Autodesk Inventor part; units mm, degrees
ref_plane "YZ Plane" through (0, 0, 0) normal (1, 0, 0) x (0, 1, 0)
ref_plane "XZ Plane" through (0, 0, 0) normal (0, 1, 0) x (-1, 0, 0)
ref_plane "XY Plane" through (0, 0, 0) normal (0, 0, 1) x (1, 0, 0)
sketch "Sketch1" plane through (0, 0, 0) normal (0, 0, 1) x (1, 0, 0)
  circle A0 centre (0, 0) radius 38.1
  circle A1 centre (0, 0) radius 31.75
  line L0 (-84.6709, -3.175) -> (-84.6709, 3.175)
  line L1 (84.6709, 3.175) -> (84.6709, -3.175)
  line L2 (84.6709, -3.175) -> (-84.6709, 3.175) construction
  line L3 (-84.6709, -3.175) -> (84.6709, 3.175) construction
  line L4 (84.6709, -3.175) -> (37.9675, -3.175)
  line L5 (-37.9675, -3.175) -> (-84.6709, -3.175)
  line L6 (-84.6709, 3.175) -> (-37.9675, 3.175)
  line L7 (37.9675, 3.175) -> (84.6709, 3.175)
  line L8 (-84.6709, 22.225) -> (-77.0509, 22.225)
  line L9 (-77.0509, 22.225) -> (-77.0509, -22.225)
  line L10 (-77.0509, -22.225) -> (-84.6709, -22.225)
  line L11 (-84.6709, -22.225) -> (-84.6709, 22.225)
  line L12 (0, 31.75) -> (0, -31.75) construction
  line L13 (84.6709, 22.225) -> (77.0509, 22.225)
  line L14 (77.0509, 22.225) -> (77.0509, -22.225)
  line L15 (77.0509, -22.225) -> (84.6709, -22.225)
  line L16 (84.6709, -22.225) -> (84.6709, 22.225)
  dimension "d0" = 76.2
  dimension "d1" = 6.35
  dimension "d2" = 169.3418
  dimension "d4" = 6.35
  dimension "d5" = 19.05
  dimension "d6" = 19.05
  dimension "d7" = 7.62
extrude "Plate1" add sketch "Sketch1" along normal blind 0.889
fillet "Corner Round1" radius 3.175 16 edges at (77.0509, -3.175, 0.4445) (77.0509, -22.225, 0.4445) (77.0509, 3.175, 0.4445) (77.0509, 22.225, 0.4445) (84.6709, -22.225, 0.4445) (84.6709, 22.225, 0.4445) (37.9675, -3.175, 0.4445) (-77.0509, -3.175, 0.4445) (-77.0509, -22.225, 0.4445) (-77.0509, 3.175, 0.4445) (-77.0509, 22.225, 0.4445) (-84.6709, -22.225, 0.4445) (-84.6709, 22.225, 0.4445) (-37.9675, 3.175, 0.4445) (-37.9675, -3.175, 0.4445) (37.9675, 3.175, 0.4445)
equation "\"d8\" = Thickness"
equation "\"BendRadius\" = Thickness"
equation "\"BendReliefWidth\" = Thickness"
equation "\"BendReliefDepth\" = 0.5 * Thickness"
equation "\"CornerReliefSize\" = 4 * Thickness"
equation "\"MinimumRemnant\" = 2 * Thickness"
equation "\"TransitionRadius\" = BendRadius"
equation "\"JacobiRadiusSize\" = Thickness"
equation "\"GapSize\" = Thickness"
properties part number "Frame" material "Aluminum 6061"
Source: CAD feature listing. Evaluate the final solid. Frame: model axes, mm. A direction names the side the tool comes from. Round coordinates to 2 decimals unless told otherwise and drop trailing zeros. Write each loop counter-clockwise with the first axis right and the second up, starting at its lowest first coordinate (ties: lowest second). Pieces come first, ordered by that corner, then holes. Notation, with made-up numbers: M 4,25.5 L 54,25.5 A21 cw 54,56.5 Z; hole C 4.5,70.25 d1. An arc over 180 degrees is marked long. Answer as a JSON object with one key per item and string values. Group by question number.
(1) Section query A-A on y = 0. Output: boundary loops of the cut face in (x, z), then the cut area to 3 significant figures.
(2) Section query B-B on x = 0. Output: boundary loops of the cut face in (y, z), then the cut area to 3 significant figures.
(3) Section query D-D on y = 15.5. Output: boundary loops of the cut face in (x, z), then the cut area to 3 significant figures.
(4) Reachability of faces 4 (the cylindrical face through (-76.096, -4.08, 0.451)), 5 (the cylindrical face through (-83.716, 21.32, 0.451)), 6 (the cylindrical face through (76.096, 4.08, 0.451)) from +Z, -Z, +X, -X, +Y, -Y: full face, straight path, thin tool, end or side. Return the list, or none.
(5) Ray query, line 1 (Y direction, x = 0, z = 0.5); line 2 (X direction, y = 9, z = 0.25); line 3 (Y direction, x = 68.5, z = 0.45) (3 decimals). Return the intervals inside material, ascending. Write a range as [from, to].
(6) Mould query, pull axis X, two halves, no side actions, for faces 1 (the cylindrical face through (-83.766, -21.27, 0.451)), 2 (the flat face through (-32, 0, 0.889)), 3 (the cylindrical face through (-0.755, 38.093, 0.438)). Classes: +X half, -X half, draft (parallel to the pull), parting line (faces both ways), or undercut.
Computed values:
{
 "1": {"outline": "M -84.67,0 L -31.75,0 L -31.75,0.89 L -84.67,0.89 Z; M 31.75,0 L 84.67,0 L 84.67,0.89 L 31.75,0.89 Z", "area": "94.1 mm^2"},
 "2": {"outline": "M -38.1,0 L -31.75,0 L -31.75,0.89 L -38.1,0.89 Z; M 31.75,0 L 38.1,0 L 38.1,0.89 L 31.75,0.89 Z", "area": "11.3 mm^2"},
 "3": {"outline": "M -84.67,0 L -77.05,0 L -77.05,0.89 L -84.67,0.89 Z; M -34.8,0 L -27.71,0 L -27.71,0.89 L -34.8,0.89 Z; M 27.71,0 L 34.8,0 L 34.8,0.89 L 27.71,0.89 Z; M 77.05,0 L 84.67,0 L 84.67,0.89 L 77.05,0.89 Z", "area": "26.2 mm^2"},
 "4": {"face 4": "+Z, -Z, -Y", "face 5": "+Z, -Z, -X, +Y", "face 6": "+Z, -Z, +Y"},
 "5": {"line 1": "[-38.1, -31.75], [31.75, 38.1]", "line 2": "[-84.67, -77.05], [-37.02, -30.45], [30.45, 37.02], [77.05, 84.67]", "line 3": "[-3.175, 3.175]"},
 "6": {"face 1": "-X half", "face 2": "draft", "face 3": "undercut"}
}
